from build123d import *

# Parameters (mm, degrees)
SKETCH_1_W            = 426
SKETCH_1_H            = 40
EXTRUDE_1_DEPTH       = 3.7
SKETCH_1_2_W          = 426
SKETCH_1_2_H          = 40
SKETCH_1_2_W_2        = 422.8
SKETCH_1_2_H_2        = 36.8
CUT_EXTRUDE_1_DEPTH   = 1.2
SKETCH_2_R            = 10.15
SKETCH_2_R_2          = 3.25
SKETCH_2_R_3          = 3.75
SKETCH_2_R_4          = 2.75
SKETCH_2_R_5          = 3
CUT_EXTRUDE_1_2_DEPTH = 10
SKETCH_4_R            = 12
CUT_EXTRUDE_2_DEPTH   = 1.7
SKETCH_2_3_R          = 6
SKETCH_2_3_R_2        = 3
SKETCH_2_3_R_3        = 6.25
SKETCH_2_3_R_4        = 3.25
CUT_EXTRUDE_2_2_DEPTH = 2.5
EXTRUDE_2_DEPTH       = 0.1
SKETCH_2_5_R          = 6.25
CUT_EXTRUDE_3_DEPTH   = 2.5


with BuildPart() as part:
    # Эскиз1 → Бобышка-Вытянуть1 (new body)
    with BuildSketch(Plane(origin=(0, 0, 0), x_dir=(1, 0, 0), z_dir=(0, 1, 0))):
        Rectangle(SKETCH_1_W, SKETCH_1_H)
    extrude(amount=EXTRUDE_1_DEPTH)

    # Эскиз1<2> → Cut-Extrude 1 (cut)
    with BuildSketch(Plane(origin=(0, 0, 0), x_dir=(1, 0, 0), z_dir=(0, 1, 0))):
        Rectangle(SKETCH_1_2_W, SKETCH_1_2_H)
        Rectangle(SKETCH_1_2_W_2, SKETCH_1_2_H_2, mode=Mode.SUBTRACT)
    extrude(amount=CUT_EXTRUDE_1_DEPTH, mode=Mode.SUBTRACT)

    # Эскиз2 → Cut-Extrude 1 2 (cut)
    with BuildSketch(Plane(origin=(0, 0, 0), x_dir=(1, 0, 0), z_dir=(0, 1, 0))):
        with Locations((-183, 0)):
            Circle(SKETCH_2_R)
        with BuildLine():
            Line((-195.35, -1.5), (-193.038550692, -1.5))
            ThreePointArc((-193.038550692, -1.5), (-193.15, 0), (-193.038550692, 1.5))
            Line((-193.038550692, 1.5), (-195.35, 1.5))
            Line((-195.35, 1.5), (-195.35, -1.5))
        make_face()
        with Locations(Location((-143, 0, 0), (0, 0, 270))):
            Circle(SKETCH_2_R_2)
        with Locations(Location((-118, 0, 0), (0, 0, 270))):
            Circle(SKETCH_2_R_3)
        with Locations(Location((-83, 0, 0), (0, 0, 270))):
            Circle(SKETCH_2_R_2)
        with Locations(Location((-58, 0, 0), (0, 0, 270))):
            Circle(SKETCH_2_R_3)
        with Locations(Location((-13, 0, 0), (0, 0, 270))):
            Circle(SKETCH_2_R_3)
        with Locations(Location((17, 0, 0), (0, 0, 270))):
            Circle(SKETCH_2_R_3)
        with Locations(Location((47, 0, 0), (0, 0, 270))):
            Circle(SKETCH_2_R_3)
        with Locations(Location((95, 0, 0), (0, 0, 270))):
            Circle(SKETCH_2_R_4)
        with Locations(Location((103, 0, 0), (0, 0, 270))):
            Circle(SKETCH_2_R_4)
        with Locations(Location((119, 0, 0), (0, 0, 270))):
            Circle(SKETCH_2_R_4)
        with Locations(Location((188, 0, 0), (0, 0, 270))):
            Circle(SKETCH_2_R_5)
        with BuildLine():
            Line((157, -9), (159, -9))
            ThreePointArc((159, -9), (160, -8), (159, -7))
            Line((159, -7), (157, -7))
            ThreePointArc((157, -7), (156, -8), (157, -9))
        make_face()
        with Locations(Location((87, 0, 0), (0, 0, 270))):
            Circle(SKETCH_2_R_4)
        with Locations(Location((111, 0, 0), (0, 0, 270))):
            Circle(SKETCH_2_R_4)
        with Locations(Location((158, 0, 0), (0, 0, 270))):
            Circle(SKETCH_2_R_3)
    extrude(amount=CUT_EXTRUDE_1_2_DEPTH, mode=Mode.SUBTRACT)

    # Эскиз4 → Cut-Extrude 2 (cut)
    with BuildSketch(Plane(origin=(0, 0, 0), x_dir=(1, 0, 0), z_dir=(0, 1, 0))):
        with Locations((-183, 0)):
            Circle(SKETCH_4_R)
    extrude(amount=CUT_EXTRUDE_2_DEPTH, mode=Mode.SUBTRACT)

    # Эскиз2<3> → Cut-Extrude 2 2 (cut)
    # profile 1 of 3: a face of its own
    with BuildSketch(Plane(origin=(0, 0, 0), x_dir=(1, 0, 0), z_dir=(0, 1, 0))):
        with Locations((188, 0)):
            Circle(SKETCH_2_3_R)
        with Locations((188, 0)):
            Circle(SKETCH_2_3_R_2, mode=Mode.SUBTRACT)
    # profile 2 of 3: a face of its own
    with BuildSketch(Plane(origin=(0, 0, 0), x_dir=(1, 0, 0), z_dir=(0, 1, 0))):
        with Locations((-83, 0)):
            Circle(SKETCH_2_3_R_3)
        with Locations((-83, 0)):
            Circle(SKETCH_2_3_R_4, mode=Mode.SUBTRACT)
    # profile 3 of 3: a face of its own
    with BuildSketch(Plane(origin=(0, 0, 0), x_dir=(1, 0, 0), z_dir=(0, 1, 0))):
        with Locations((-143, 0)):
            Circle(SKETCH_2_3_R_3)
        with Locations((-143, 0)):
            Circle(SKETCH_2_3_R_4, mode=Mode.SUBTRACT)
    extrude(amount=CUT_EXTRUDE_2_2_DEPTH, mode=Mode.SUBTRACT)

    # Эскиз3 → Бобышка-Вытянуть2 (add)
    # profile 1 of 6: a face of its own
    with BuildSketch(Plane(origin=(0, 0, 0), x_dir=(1, 0, 0), z_dir=(0, 1, 0))):
        with BuildLine():
            Line((-152, -15), (-109, -15))
            ThreePointArc((-109, -15), (-104.757359313, -13.242640687), (-103, -9))
            Line((-103, -9), (-103, 9))
            ThreePointArc((-103, 9), (-104.757359313, 13.242640687), (-109, 15))
            Line((-109, 15), (-152, 15))
            ThreePointArc((-152, 15), (-156.242640687, 13.242640687), (-158, 9))
            Line((-158, 9), (-158, -9))
            ThreePointArc((-158, -9), (-156.242640687, -13.242640687), (-152, -15))
        make_face()
        with BuildLine():
            Line((-152, -13.5), (-109, -13.5))
            ThreePointArc((-109, -13.5), (-105.818019485, -12.181980515), (-104.5, -9))
            Line((-104.5, -9), (-104.5, 9))
            ThreePointArc((-104.5, 9), (-105.818019485, 12.181980515), (-109, 13.5))
            Line((-109, 13.5), (-152, 13.5))
            ThreePointArc((-152, 13.5), (-155.181980515, 12.181980515), (-156.5, 9))
            Line((-156.5, 9), (-156.5, -9))
            ThreePointArc((-156.5, -9), (-155.181980515, -12.181980515), (-152, -13.5))
        make_face(mode=Mode.SUBTRACT)
    # profile 2 of 6: a face of its own
    with BuildSketch(Plane(origin=(0, 0, 0), x_dir=(1, 0, 0), z_dir=(0, 1, 0))):
        with BuildLine():
            Line((-22, -15), (56, -15))
            ThreePointArc((56, -15), (60.242640687, -13.242640687), (62, -9))
            Line((62, -9), (62, 9))
            ThreePointArc((62, 9), (60.242640687, 13.242640687), (56, 15))
            Line((56, 15), (-22, 15))
            ThreePointArc((-22, 15), (-26.242640687, 13.242640687), (-28, 9))
            Line((-28, 9), (-28, -9))
            ThreePointArc((-28, -9), (-26.242640687, -13.242640687), (-22, -15))
        make_face()
        with BuildLine():
            Line((-22, -13.5), (56, -13.5))
            ThreePointArc((56, -13.5), (59.181980515, -12.181980515), (60.5, -9))
            Line((60.5, -9), (60.5, 9))
            ThreePointArc((60.5, 9), (59.181980515, 12.181980515), (56, 13.5))
            Line((56, 13.5), (-22, 13.5))
            ThreePointArc((-22, 13.5), (-25.181980515, 12.181980515), (-26.5, 9))
            Line((-26.5, 9), (-26.5, -9))
            ThreePointArc((-26.5, -9), (-25.181980515, -12.181980515), (-22, -13.5))
        make_face(mode=Mode.SUBTRACT)
    # profile 3 of 6: a face of its own
    with BuildSketch(Plane(origin=(0, 0, 0), x_dir=(1, 0, 0), z_dir=(0, 1, 0))):
        with BuildLine():
            Line((83, -15), (123, -15))
            ThreePointArc((123, -15), (127.242640687, -13.242640687), (129, -9))
            Line((129, -9), (129, 9))
            ThreePointArc((129, 9), (127.242640687, 13.242640687), (123, 15))
            Line((123, 15), (83, 15))
            ThreePointArc((83, 15), (78.757359313, 13.242640687), (77, 9))
            Line((77, 9), (77, -9))
            ThreePointArc((77, -9), (78.757359313, -13.242640687), (83, -15))
        make_face()
        with BuildLine():
            Line((83, -13.5), (123, -13.5))
            ThreePointArc((123, -13.5), (126.181980515, -12.181980515), (127.5, -9))
            Line((127.5, -9), (127.5, 9))
            ThreePointArc((127.5, 9), (126.181980515, 12.181980515), (123, 13.5))
            Line((123, 13.5), (83, 13.5))
            ThreePointArc((83, 13.5), (79.818019485, 12.181980515), (78.5, 9))
            Line((78.5, 9), (78.5, -9))
            ThreePointArc((78.5, -9), (79.818019485, -12.181980515), (83, -13.5))
        make_face(mode=Mode.SUBTRACT)
    # profile 4 of 6: a face of its own
    with BuildSketch(Plane(origin=(0, 0, 0), x_dir=(1, 0, 0), z_dir=(0, 1, 0))):
        with BuildLine():
            Line((146, -15), (196, -15))
            ThreePointArc((196, -15), (200.242640687, -13.242640687), (202, -9))
            Line((202, -9), (202, 9))
            ThreePointArc((202, 9), (200.242640687, 13.242640687), (196, 15))
            Line((196, 15), (146, 15))
            ThreePointArc((146, 15), (141.757359313, 13.242640687), (140, 9))
            Line((140, 9), (140, -9))
            ThreePointArc((140, -9), (141.757359313, -13.242640687), (146, -15))
        make_face()
        with BuildLine():
            Line((146, -13.5), (196, -13.5))
            ThreePointArc((196, -13.5), (199.181980515, -12.181980515), (200.5, -9))
            Line((200.5, -9), (200.5, 9))
            ThreePointArc((200.5, 9), (199.181980515, 12.181980515), (196, 13.5))
            Line((196, 13.5), (146, 13.5))
            ThreePointArc((146, 13.5), (142.818019485, 12.181980515), (141.5, 9))
            Line((141.5, 9), (141.5, -9))
            ThreePointArc((141.5, -9), (142.818019485, -12.181980515), (146, -13.5))
        make_face(mode=Mode.SUBTRACT)
    # profile 5 of 6: a face of its own
    with BuildSketch(Plane(origin=(0, 0, 0), x_dir=(1, 0, 0), z_dir=(0, 1, 0))):
        with BuildLine():
            Line((-92, -15), (-49, -15))
            ThreePointArc((-49, -15), (-44.757359313, -13.242640687), (-43, -9))
            Line((-43, -9), (-43, 9))
            ThreePointArc((-43, 9), (-44.757359313, 13.242640687), (-49, 15))
            Line((-49, 15), (-92, 15))
            ThreePointArc((-92, 15), (-96.242640687, 13.242640687), (-98, 9))
            Line((-98, 9), (-98, -9))
            ThreePointArc((-98, -9), (-96.242640687, -13.242640687), (-92, -15))
        make_face()
        with BuildLine():
            Line((-92, -13.5), (-49, -13.5))
            ThreePointArc((-49, -13.5), (-45.818019485, -12.181980515), (-44.5, -9))
            Line((-44.5, -9), (-44.5, 9))
            ThreePointArc((-44.5, 9), (-45.818019485, 12.181980515), (-49, 13.5))
            Line((-49, 13.5), (-92, 13.5))
            ThreePointArc((-92, 13.5), (-95.181980515, 12.181980515), (-96.5, 9))
            Line((-96.5, 9), (-96.5, -9))
            ThreePointArc((-96.5, -9), (-95.181980515, -12.181980515), (-92, -13.5))
        make_face(mode=Mode.SUBTRACT)
    # profile 6 of 6: a face of its own
    with BuildSketch(Plane(origin=(0, 0, 0), x_dir=(1, 0, 0), z_dir=(0, 1, 0))):
        with BuildLine():
            Line((-197, -15), (-169, -15))
            ThreePointArc((-169, -15), (-164.757359313, -13.242640687), (-163, -9))
            Line((-163, -9), (-163, 9))
            ThreePointArc((-163, 9), (-164.757359313, 13.242640687), (-169, 15))
            Line((-169, 15), (-197, 15))
            ThreePointArc((-197, 15), (-201.242640687, 13.242640687), (-203, 9))
            Line((-203, 9), (-203, -9))
            ThreePointArc((-203, -9), (-201.242640687, -13.242640687), (-197, -15))
        make_face()
        with BuildLine():
            Line((-197, -13.5), (-169, -13.5))
            ThreePointArc((-169, -13.5), (-165.818019485, -12.181980515), (-164.5, -9))
            Line((-164.5, -9), (-164.5, 9))
            ThreePointArc((-164.5, 9), (-165.818019485, 12.181980515), (-169, 13.5))
            Line((-169, 13.5), (-197, 13.5))
            ThreePointArc((-197, 13.5), (-200.181980515, 12.181980515), (-201.5, 9))
            Line((-201.5, 9), (-201.5, -9))
            ThreePointArc((-201.5, -9), (-200.181980515, -12.181980515), (-197, -13.5))
        make_face(mode=Mode.SUBTRACT)
    extrude(amount=-EXTRUDE_2_DEPTH)

    # Эскиз2<5> → Вырез-Вытянуть3 (cut)
    with BuildSketch(Plane(origin=(0, 0, 0), x_dir=(1, 0, 0), z_dir=(0, 1, 0))):
        with Locations(Location((-13, 0, 0), (0, 0, 270))):
            Circle(SKETCH_2_5_R)
        with Locations(Location((17, 0, 0), (0, 0, 270))):
            Circle(SKETCH_2_5_R)
        with Locations(Location((47, 0, 0), (0, 0, 270))):
            Circle(SKETCH_2_5_R)
        with Locations(Location((-118, 0, 0), (0, 0, 270))):
            Circle(SKETCH_2_5_R)
        with Locations(Location((-58, 0, 0), (0, 0, 270))):
            Circle(SKETCH_2_5_R)
    extrude(amount=CUT_EXTRUDE_3_DEPTH, mode=Mode.SUBTRACT)


solid = part.part
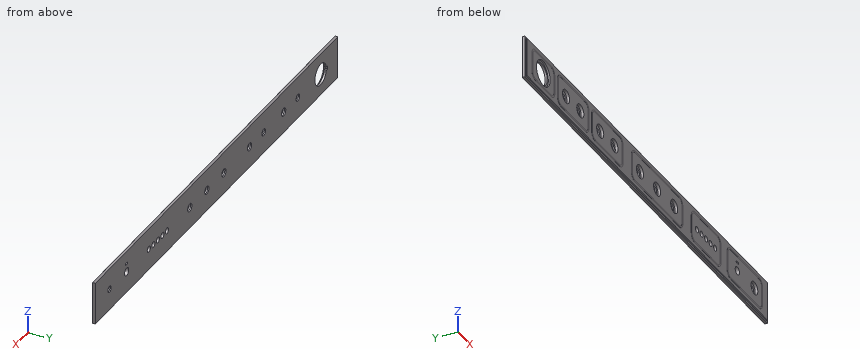
Model file for the job. Use its own axes, mm. Give positions to 0.01 mm unless a question says otherwise; leave off trailing zeros. Loops run counter-clockwise (first coordinate to the right, second up) from the corner with the lowest first, then second, coordinate; pieces in that order, holes last.
Item 1: Drill centre lines: line 1 along Z through (x, y) = (-184, 3.25); line 2 along Z through (x, y) = (-58, 3.05); line 3 along X through (y, z) = (3.4, 7.5). Where is each one in solid material? Low to high.
Check values:
line 1: z = -20 to -10.1, 10.1 to 20
line 2: z = -20 to -3.75, 3.75 to 20
line 3: x = -213 to -189.84, -176.16 to 156.13, 159.87 to 213
Item 2: Slice it at A-A (x = -183). Write the cut outline in (y, z), plus the area to 3 significant figures.
Check values:
outline: (-0.1, -15) - (0, -15) - (0, -18.4) - (1.2, -18.4) - (1.2, -20) - (3.7, -20) - (3.7, -10.15) - (1.7, -10.15) - (1.7, -12) - (0, -12) - (0, -13.5) - (-0.1, -13.5) - close; (-0.1, 13.5) - (0, 13.5) - (0, 12) - (1.7, 12) - (1.7, 10.15) - (3.7, 10.15) - (3.7, 20) - (1.2, 20) - (1.2, 18.4) - (0, 18.4) - (0, 15) - (-0.1, 15) - close
area: 63.1 mm2
Item 3: Slice it at B-B (y = 0.6). Give the number of separate pieces and of enclosed holes in the cut face, plus the area to 3 significant figures.
Check values:
separate pieces: 1
enclosed holes: 16
area: 14,000 mm2
Item 4: Drop flat-ended pins along their axis: P1, Ø1.3, axis at y = 0.5, z = -4, coming from the +X side; P2, Ø4, axis at x = 33, z = -9.5, coming from the -Y side; P3, Ø1, axis at y = 0.5, z = 1.5, coming from the -X side. Give the stop position or say it passes through.
Check values:
P1: stops at x = 211.4
P2: stops at y = 0
P3: stops at x = -211.4
Item 5: Slice it at C-C (x = 0.5). Write the cut outline in (y, z).
Check values:
outline: (-0.1, -15) - (0, -15) - (0, -18.4) - (1.2, -18.4) - (1.2, -20) - (3.7, -20) - (3.7, 20) - (1.2, 20) - (1.2, 18.4) - (0, 18.4) - (0, 15) - (-0.1, 15) - (-0.1, 13.5) - (0, 13.5) - (0, -13.5) - (-0.1, -13.5) - close
Item 6: Slice it at D-D (x = 47). Write the cut outline in (y, z), plus the area to 3 significant figures.
Check values:
outline: (-0.1, -15) - (0, -15) - (0, -18.4) - (1.2, -18.4) - (1.2, -20) - (3.7, -20) - (3.7, -3.75) - (2.5, -3.75) - (2.5, -6.25) - (0, -6.25) - (0, -13.5) - (-0.1, -13.5) - close; (-0.1, 13.5) - (0, 13.5) - (0, 6.25) - (2.5, 6.25) - (2.5, 3.75) - (3.7, 3.75) - (3.7, 20) - (1.2, 20) - (1.2, 18.4) - (0, 18.4) - (0, 15) - (-0.1, 15) - close
area: 104 mm2
